Part model, mm, in its own coordinate system. Round coordinates to 2 decimals unless told otherwise and drop trailing zeros. Order: outer loops, then holes, each group sorted by start corner. A loop starts at its lowest first (then second) coordinate and runs counter-clockwise, first axis right, second up. Notation, with made-up numbers: (-22.75, 89.5) -> (-3.75, 89.5) arc R19 cw to (-3.75, 125.5) -> close; hole circle Ø8 at (38.25, -26). An arc over 180 degrees is marked (long way). Answer as a JSON object with one key per item and string values. Group by question number.
Autodesk Inventor part; units mm, degrees
ref_plane "YZ Plane" through (0, 0, 0) normal (1, 0, 0) x (0, 1, 0)
ref_plane "XZ Plane" through (0, 0, 0) normal (0, 1, 0) x (-1, 0, 0)
ref_plane "XY Plane" through (0, 0, 0) normal (0, 0, 1) x (1, 0, 0)
sketch "Sketch1" plane through (0, 0, 0) normal (0, 1, 0) x (-1, 0, 0)
  line L0 (30, 35) -> (-30, 35)
  line L1 (-30, 35) -> (-30, -35)
  line L2 (-30, -35) -> (30, -35)
  line L3 (30, -35) -> (30, 35)
  line L4 (30, 35) -> (-30, -35) construction
  line L5 (-30, 35) -> (30, -35) construction
  point P0 (0, 0)
  dimension "d0" = 60
  dimension "d1" = 70
extrude "Extrusion1" add sketch "Sketch1" along normal blind 2
sketch "Sketch2" plane through (0, 2, 0) normal (0, 1, 0) x (1, 0, 0)
  circle A0 centre (-23.5, -28.5) radius 2
  line L0 (-30, 35) -> (-30, -35)
  line L1 (-30, -35) -> (30, -35)
  point P0 (0, 0)
  dimension "d4" = 4
  dimension "d5" = 6.5
  dimension "d6" = 6.5
extrude "Extrusion2" cut sketch "Sketch2" against normal blind 2
mirror "Mirror1" about plane through (0, 0, 0) normal (0, 0, 1) of "Extrusion2"
mirror "Mirror2" about plane through (0, 0, 0) normal (1, 0, 0) of "Extrusion2", "Mirror1"
fillet "Fillet1" radius 3 4 edges at (-30, 1, 35) (-30, 1, -35) (30, 1, -35) (30, 1, 35)
properties part number "Kraicka_senzory_vrchnak"
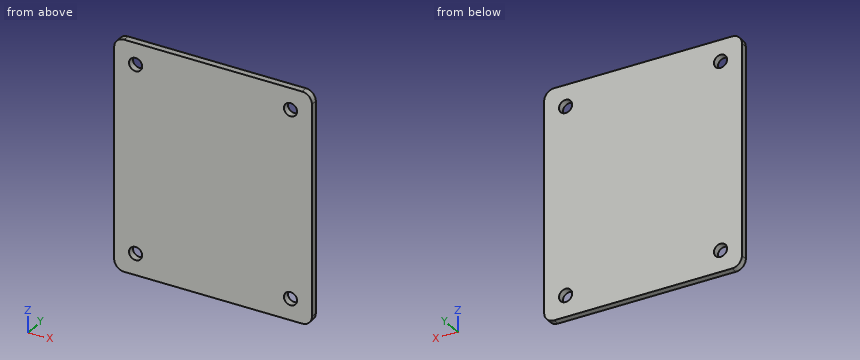
Q1. Band-saw the part on A-A (z = 28.5). List the corners of the cut face in (x, y), plus the area to 3 significant figures.
Q2. Wall check: line 1 (Z direction, x = 23.5, y = 1.35); line 2 (X direction, y = 0.8, z = 28.5); line 3 (Z direction, x = 24, y = 1.1). Give the ranges that are in metal, low to high. Write a range as [from, to].
Q3. Drop a flat-ended pin along its axis: pin 1 Ø6.5 at (x, z) = (-23.5, 28.5) entering from +Y. Give the stop position or say it passes through.
Q4. Band-saw the part on B-B (x = -23.5). List the corners of the cut face in (y, z), plus the area to 3 significant figures.
Completed:
{
 "1": {"outline": "(-30, 0) -> (-25.5, 0) -> (-25.5, 2) -> (-30, 2) -> close; (-21.5, 0) -> (21.5, 0) -> (21.5, 2) -> (-21.5, 2) -> close; (25.5, 0) -> (30, 0) -> (30, 2) -> (25.5, 2) -> close", "area": "104 mm2"},
 "2": {"line 1": "[-35, -30.5], [-26.5, 26.5], [30.5, 35]", "line 2": "[-30, -25.5], [-21.5, 21.5], [25.5, 30]", "line 3": "[-35, -30.44], [-26.56, 26.56], [30.44, 35]"},
 "3": {"pin 1": "y = 2"},
 "4": {"outline": "(0, -35) -> (2, -35) -> (2, -30.5) -> (0, -30.5) -> close; (0, -26.5) -> (2, -26.5) -> (2, 26.5) -> (0, 26.5) -> close; (0, 30.5) -> (2, 30.5) -> (2, 35) -> (0, 35) -> close", "area": "124 mm2"}
}
